Geometry: final body of the model. Coordinates: model frame, mm. Face numbers are marked on the shaded views. A direction names the side the tool comes from. Round coordinates to 2 decimals unless told otherwise and drop trailing zeros. Loops run counter-clockwise (first coordinate to the right, second up) from the corner with the lowest first, then second, coordinate; pieces in that order, holes last. Notation, with made-up numbers: (-19.5, 11.25) - (10.5, 11.25) arc R5 cw to (10.5, 16.25) - close; hole circle Ø10 at (85, 89.25). An arc over 180 degrees is marked (long way). Answer in a Markdown table with one row per item. Add a question column.
from build123d import *

# Parameters (mm, degrees)
EXTRUDE_1_DEPTH     = 10
SKETCH_2_R          = 2.5
CUT_EXTRUDE_1_DEPTH = 112.943065886
SKETCH_3_R          = 1.5
CUT_EXTRUDE_2_DEPTH = 92.172912644
SKETCH_4_W          = 50
SKETCH_4_H          = 55
CUT_EXTRUDE_3_DEPTH = 92.172912644
CHAMFER_1_SIZE      = 2


with BuildPart() as part:
    # 草图1 → 凸台-拉伸1 (new body)
    with BuildSketch(Plane(origin=(0, 0, 0), x_dir=(1, 0, 0), z_dir=(0, 1, 0))):
        with BuildLine():
            Line((0, 37.5), (82.5, 37.5))
            Line((82.5, 37.5), (82.5, -37.5))
            Line((82.5, -37.5), (0, -37.5))
            ThreePointArc((0, -37.5), (-37.5, 0), (0, 37.5))
        make_face()
    extrude(amount=EXTRUDE_1_DEPTH)

    # 草图2 → 切除-拉伸1 (cut, through all)
    with BuildSketch(Plane.XY.offset(37.5)):
        with Locations(Location((2.5, 5, 0), (0, 0, 180))):
            Circle(SKETCH_2_R)
    extrude(amount=-CUT_EXTRUDE_1_DEPTH, mode=Mode.SUBTRACT)

    # 草图3 → 切除-拉伸2 (cut, through all)
    with BuildSketch(Plane(origin=(0, 10, 0), x_dir=(1, 0, 0), z_dir=(0, 1, 0))):
        with Locations(Location((-27.5, 20, 0), (0, 0, 270))):
            Circle(SKETCH_3_R)
        with Locations(Location((-27.5, -20, 0), (0, 0, 270))):
            Circle(SKETCH_3_R)
        with Locations(Location((77.5, 32.5, 0), (0, 0, 270))):
            Circle(SKETCH_3_R)
        with Locations(Location((77.5, -32.5, 0), (0, 0, 270))):
            Circle(SKETCH_3_R)
    extrude(amount=-CUT_EXTRUDE_2_DEPTH, mode=Mode.SUBTRACT)

    # 草图4 → 切除-拉伸3 (cut, through all)
    with BuildSketch(Plane(origin=(0, 10, 0), x_dir=(1, 0, 0), z_dir=(0, 1, 0))):
        with Locations((47.5, 0)):
            Rectangle(SKETCH_4_W, SKETCH_4_H)
    extrude(amount=-CUT_EXTRUDE_3_DEPTH, mode=Mode.SUBTRACT)

    # 倒角1
    chamfer_1_edges = [part.edges().sort_by_distance(p)[0] for p in [
        (82.5, 5, -37.5),
        (82.5, 5, 37.5),
    ]]
    chamfer(chamfer_1_edges, length=CHAMFER_1_SIZE)


solid = part.part
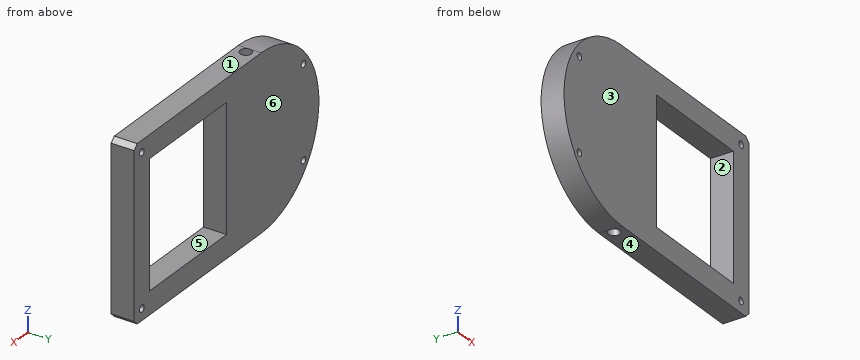
1) Reachability of the marked faces 5 and 6 from +Z, -Z, +X, -X, +Y, -Y: full face, straight path, thin tool, end or side. Return the list, or none.
2) Pull-direction query (Z, two-part tool) for the marked faces 1, 2, 3 and 4; classes: pulls with the +Z half, pulls with the -Z half, needs draft (parallel to the pull), parting line crosses it, or undercut.
3) Section A-A, the plane x = 45.5. Return the cut outline in (y, z), and give its area (3 significant figures).
4) Section B-B, the plane z = -20. Return the cut outline in (x, y), and give its area (3 significant figures).
5) Contact query for flat-ended pins moving along their axis: pin 1 Ø1 at (x, y) = (-22.5, 7.5) entering from -Z; pin 2 Ø2 at (y, z) = (9, -4.5) entering from -X. Output: stop coordinate, or through.
6) Material intervals for line 1 along Z through (x, y) = (77.5, 4.25); line 2 along Z through (x, y) = (44, 6.5); line 3 along X through (y, z) = (5, 5), sorted ascending. Write a range as from..to.
7) Section C-C, the plane x = 77.5. Return the cut outline in (y, z).
8) Section D-D, the plane z = -32.5. Return the cut outline in (x, y), and give its area (3 significant figures).
Evaluation:
| question | item | result |
|---|---|---|
| 1 | face 5 | +Y, -Y |
| 1 | face 6 | +Z, -Z, +X, -X, +Y |
| 2 | face 1 | pulls with the +Z half |
| 2 | face 2 | undercut |
| 2 | face 3 | needs draft |
| 2 | face 4 | pulls with the -Z half |
| 3 | outline | (0, -37.5) - (10, -37.5) - (10, -27.5) - (0, -27.5) - close; (0, 27.5) - (10, 27.5) - (10, 37.5) - (0, 37.5) - close |
| 3 | area | 200 mm² |
| 4 | outline | (-31.72, 0) - (-29, 0) - (-29, 10) - (-31.72, 10) - close; (-26, 0) - (22.5, 0) - (22.5, 10) - (-26, 10) - close; (72.5, 0) - (82.5, 0) - (82.5, 10) - (72.5, 10) - close; hole circle Ø5 at (2.5, 5) |
| 4 | area | 593 mm² |
| 5 | pin 1 | stops at z = -30.37 |
| 5 | pin 2 | stops at x = -37.34 |
| 6 | line 1 | z = -37.5..-34, -31..31, 34..37.5 |
| 6 | line 2 | z = -37.5..-27.5, 27.5..37.5 |
| 6 | line 3 | x = -37.17..0, 5..22.5, 72.5..82.5 |
| 7 | outline | (0, -37.5) - (10, -37.5) - (10, -34) - (0, -34) - close; (0, -31) - (10, -31) - (10, 31) - (0, 31) - close; (0, 34) - (10, 34) - (10, 37.5) - (0, 37.5) - close |
| 8 | outline | (-18.71, 0) - (76, 0) - (76, 10) - (-18.71, 10) - close; (79, 0) - (82.5, 0) - (82.5, 10) - (79, 10) - close; hole circle Ø5 at (2.5, 5) |
| 8 | area | 962 mm² |
